Part model, mm, in its own coordinate system. A direction names the side the tool comes from. Give positions to 0.01 mm unless a question says otherwise; leave off trailing zeros. Order: outer loops, then holes, each group sorted by start corner. A loop starts at its lowest first (then second) coordinate and runs counter-clockwise, first axis right, second up.
1. Drop a flat-ended pin along its axis: pin 1 Ø0.6 at (y, z) = (-21.5, -0.5) entering from +X. Give the stop position or say it passes through.
2. Mould opens along X. For faces 4 (the cylindrical face through (-40.18, -50.29, -0.55)), 5 (the cylindrical face through (108.859, -58.797, 2.465)), 6 (the flat face through (29, 50, 2)) say: +X half, -X half, draft (parallel to the pull), parting line (faces both ways), or undercut.
3. Which spindle directions (+Z, -Z, +X, -X, +Y, -Y) get a long thin tool onto all of the face, cutting with end or side? Do faces 1 (the cylindrical face through (-39, -49.08, 0.25)), 2 (the flat face through (85, -6, 3)), 3 (the cylindrical face through (-48.797, -58.859, 2.465)). Say none if no direction does.
4. Probe line 1 (Y direction, x = -45, z = 2.7); line 2 (Y direction, x = 54.5, z = 1.15); line 3 (Y direction, x = 5.5, z = -0.2). List the from-to ranges inside material, lowest first.
5. Slice it at C-C on z = 3.6. List the corners of the cut face in (x, y), and give its area (3 significant figures).
Autodesk Fusion 360 part; units mm, degrees
sketch "Sketch2" plane through (0, 0, 0) normal (0, 0, 1) x (1, 0, 0)
  line L0 (-46, 50) -> (106, 50)
  line L1 (110, 46) -> (110, -56)
  line L2 (106, -60) -> (-46, -60)
  line L3 (-50, -56) -> (-50, 46)
  circle A0 centre (-45, 45) radius 2
  line L4 (30, -60) -> (30, 50) construction
  line L5 (-50, -5) -> (110, -5) construction
  arc A1 (-46, 50) -> (-50, 46) centre (-46, 46) ccw
  circle A2 centre (105, 45) radius 2
  arc A3 (110, 46) -> (106, 50) centre (106, 46) ccw
  circle A4 centre (105, -55) radius 2
  arc A5 (106, -60) -> (110, -56) centre (106, -56) ccw
  circle A6 centre (-45, -55) radius 2
  arc A7 (-50, -56) -> (-46, -60) centre (-46, -56) ccw
  point P0 (-50, 50)
  point P1 (110, 50)
  dimension "d3" = 4
  dimension "d4" = 5
  dimension "d5" = 5
  dimension "d6" = 4
  dimension "d63" = 160
  dimension "d64" = 110
extrude "Extrude1" add sketch "Sketch2" along normal blind 5
sketch "Sketch3" plane through (0, 0, 0) normal (0, 0, -1) x (1, 0, 0)
  circle A0 centre (105, 55) radius 2
  circle A1 centre (-45, 55) radius 2
  circle A2 centre (-45, -45) radius 2
  circle A3 centre (105, -45) radius 2
  arc A4 (-50, -46) -> (-46, -50) centre (-46, -46) ccw
  line L0 (-46, -50) -> (106, -50)
  arc A5 (106, -50) -> (110, -46) centre (106, -46) ccw
  line L1 (110, -46) -> (110, 56)
  arc A6 (110, 56) -> (106, 60) centre (106, 56) ccw
  line L2 (106, 60) -> (-46, 60)
  arc A7 (-46, 60) -> (-50, 56) centre (-46, 56) ccw
  line L3 (-50, 56) -> (-50, -46)
  line L4 (30, 60) -> (30, -50) construction
  line L5 (110, 5) -> (-50, 5) construction
  line L6 (101.7902, -41.7902) -> (-41.7901, -41.7902) construction
  line L7 (-41.7901, -41.7902) -> (-41.7901, 51.7901) construction
  line L8 (-41.7901, 51.7901) -> (101.7902, 51.7901) construction
  line L9 (101.7902, 51.7901) -> (101.7902, -41.7902) construction
  line L10 (101.7902, -41.7902) -> (-41.7901, 51.7901) construction
  line L11 (-41.7901, -41.7902) -> (101.7902, 51.7901) construction
  line L12 (95.2151, -42.8152) -> (-35.2152, -42.8152)
  line L13 (-42.8152, -35.2152) -> (-42.8152, 45.2151)
  line L14 (-35.2151, 52.8151) -> (95.2151, 52.8151)
  line L15 (102.8152, 45.2151) -> (102.8152, -35.2152)
  line L16 (88.9278, -33.6958) -> (-42.8152, 52.8151) construction
  line L17 (-37.4412, -35.28) -> (85.6746, 38.2522) construction
  line L18 (-40.7652, -35.2152) -> (-40.7652, 45.2152)
  line L19 (-35.2152, 50.7652) -> (95.2152, 50.7652)
  line L20 (100.7652, 45.2152) -> (100.7652, -35.2152)
  line L21 (98.2241, -39.1218) -> (-40.7652, 50.7652) construction
  line L22 (-34.7613, -32.5014) -> (82.9436, 35.6581) construction
  arc A8 (-35.2152, 50.7652) -> (-40.7652, 45.2152) centre (-35.2152, 45.2152) ccw
  arc A9 (-35.2151, 52.8151) -> (-42.8152, 45.2151) centre (-35.2152, 45.2151) ccw
  arc A10 (100.7652, 45.2152) -> (95.2152, 50.7652) centre (95.2152, 45.2152) ccw
  arc A11 (102.8152, 45.2151) -> (95.2151, 52.8151) centre (95.2152, 45.2151) ccw
  arc A12 (-40.7652, -35.2152) -> (-35.2152, -40.7652) centre (-35.2152, -35.2152) ccw
  arc A13 (-42.8152, -35.2152) -> (-35.2152, -42.8152) centre (-35.2152, -35.2152) ccw
  arc A14 (95.2152, -40.7652) -> (100.7652, -35.2152) centre (95.2152, -35.2152) ccw
  arc A15 (95.2151, -42.8152) -> (102.8151, -35.2152) centre (95.2151, -35.2152) ccw
  line L23 (95.2152, -40.7652) -> (-35.2152, -40.7652)
  point P0 (30, 5)
  point P1 (30, 5)
  point P2 (30, 5)
  point P3 (30, 5)
  point P4 (30, 5)
  dimension "d25" = 143.5803
  dimension "d27" = 93.5803
  dimension "d28" = 1.025
  dimension "d29" = 1.025
  dimension "d30" = 1.025
  dimension "d31" = 1.025
  dimension "d44" = 5.55
  dimension "d45" = 7.6
extrude "Extrude4" add sketch "Sketch3" along normal blind 0.8 contours L12 L13 L14 L15 A9 A11 A13 A15
draft "Draft3" angle 10 neutral plane through (0, 0, -0.8) pull (0, 0, -1) 16 faces at (8.2616, -50.7652, -0.5333) (98.4345, -49.736, -0.5333) (100.7652, -18.4051, -0.5333) (96.5236, 40.6087, -0.5333) (8.2616, 40.7652, -0.5333) (-36.2655, 40.6649, -0.5333) (-40.7652, 8.4051, -0.2667) (-39.736, -48.4345, -0.5333) (-42.8152, 8.4051, -0.5333) (-41.1892, 39.9132, -0.5333) (8.2616, 42.8152, -0.2667) (101.7969, 39.0152, -0.5333) (102.8152, -18.405, -0.5333) (97.0069, -52.6009, -0.5333) (8.2616, -52.8151, -0.2667) (-42.3972, -47.7009, -0.5333)
sketch "Sketch5" plane through (0, 0, -0.8) normal (0, 0, -1) x (1, 0, 0)
  line L0 (-35.2152, 50.7652) -> (95.2152, 50.7652)
  line L1 (100.7652, 45.2152) -> (100.7652, -35.2152)
  line L2 (95.2152, -40.7652) -> (-35.2152, -40.7652)
  line L3 (-40.7652, -35.2152) -> (-40.7652, 45.2152)
  line L4 (95.2151, 52.8151) -> (-35.2151, 52.8151)
  line L5 (-42.8152, 45.2151) -> (-42.8152, -35.2152)
  line L6 (-35.2152, -42.8152) -> (95.2151, -42.8152)
  line L7 (102.8151, -35.2152) -> (102.8152, 45.2151)
  line L8 (30, 52.8151) -> (30, -42.8152) construction
  line L9 (102.8151, 5) -> (-42.8152, 5) construction
  line L10 (101.7901, -41.7902) -> (-41.7902, -41.7902) construction
  line L11 (-41.7902, -41.7902) -> (-41.7902, 51.7901) construction
  line L12 (-41.7902, 51.7901) -> (101.7901, 51.7901) construction
  line L13 (101.7901, 51.7901) -> (101.7901, -41.7902) construction
  line L14 (101.7901, -41.7902) -> (-41.7902, 51.7901) construction
  line L15 (-41.7902, -41.7902) -> (101.7901, 51.7901) construction
  line L16 (95.2151, -42.3152) -> (-35.2151, -42.3152)
  line L17 (-42.3151, -35.2152) -> (-42.3151, 45.2151)
  line L18 (-35.2151, 52.3151) -> (95.2151, 52.3151)
  line L19 (102.3151, 45.2151) -> (102.3151, -35.2152)
  line L20 (89.0725, -33.6506) -> (-42.3151, 52.3151) construction
  line L21 (-42.3151, -42.3152) -> (89.0725, 43.6506) construction
  line L22 (95.2151, -41.2652) -> (-35.2151, -41.2652)
  line L23 (-41.2651, -35.2152) -> (-41.2651, 45.2151)
  line L24 (101.2651, 45.2151) -> (101.2651, -35.2152)
  line L25 (88.0406, -32.6798) -> (-41.2651, 51.2651) construction
  line L26 (-41.2651, -41.2652) -> (88.0406, 42.6798) construction
  arc A0 (100.7652, 45.2152) -> (95.2152, 50.7652) centre (95.2152, 45.2152) ccw
  arc A1 (95.2152, -40.7652) -> (100.7652, -35.2152) centre (95.2152, -35.2152) ccw
  arc A2 (-40.7652, -35.2152) -> (-35.2152, -40.7652) centre (-35.2152, -35.2152) ccw
  arc A3 (-35.2152, 50.7652) -> (-40.7652, 45.2152) centre (-35.2152, 45.2152) ccw
  arc A4 (-42.8152, -35.2152) -> (-35.2152, -42.8152) centre (-35.2152, -35.2152) ccw
  arc A5 (95.2151, -42.8152) -> (102.8151, -35.2152) centre (95.2152, -35.2152) ccw
  arc A6 (102.8152, 45.2151) -> (95.2151, 52.8152) centre (95.2152, 45.2152) ccw
  arc A7 (-35.2151, 52.8151) -> (-42.8151, 45.2151) centre (-35.2152, 45.2152) ccw
  arc A8 (-35.2151, 51.2651) -> (-41.2651, 45.2151) centre (-35.2151, 45.2151) ccw
  arc A9 (-35.2151, 52.3151) -> (-42.3151, 45.2151) centre (-35.2151, 45.2151) ccw
  arc A10 (101.2651, 45.2151) -> (95.2151, 51.2651) centre (95.2151, 45.2151) ccw
  arc A11 (102.3151, 45.2151) -> (95.2151, 52.3151) centre (95.2151, 45.2151) ccw
  line L27 (-35.2151, 51.2651) -> (95.2151, 51.2651)
  arc A12 (95.2151, -41.2652) -> (101.2651, -35.2152) centre (95.2151, -35.2152) ccw
  arc A13 (95.2151, -42.3152) -> (102.3151, -35.2152) centre (95.2151, -35.2152) ccw
  arc A14 (-41.2651, -35.2152) -> (-35.2151, -41.2652) centre (-35.2151, -35.2152) ccw
  arc A15 (-42.3151, -35.2152) -> (-35.2151, -42.3152) centre (-35.2151, -35.2152) ccw
  point P0 (30, 5)
  point P1 (30, 5)
  point P2 (30, 5)
  dimension "d36" = 143.5803
  dimension "d37" = 93.5803
  dimension "d38" = 0.525
  dimension "d39" = 0.525
  dimension "d40" = 0.525
  dimension "d41" = 0.525
  dimension "d50" = 6.05
  dimension "d51" = 7.1
extrude "Extrude6" cut sketch "Sketch5" against normal blind 0.5 contours L16 L17 L18 L19 A9 A11 A13 A15
extrude "Extrude7" cut 1 faces at (51.7384, -20.208, 0) along direction (0, 0, 1) blind 0.5
sketch "Sketch6" plane through (0, 0, 0.5) normal (0, 0, -1) x (1, 0, 0)
  line L0 (95.2152, 50.6241) -> (-35.2152, 50.6241)
  arc A0 (-35.2152, 50.6241) -> (-40.6241, 45.2152) centre (-35.2152, 45.2152) ccw
  line L1 (-40.6241, 45.2152) -> (-40.6241, -35.2152)
  arc A1 (-40.6241, -35.2152) -> (-35.2152, -40.6241) centre (-35.2152, -35.2152) ccw
  line L2 (-35.2152, -40.6241) -> (95.2152, -40.6241)
  arc A2 (95.2152, -40.6241) -> (100.6241, -35.2152) centre (95.2152, -35.2152) ccw
  line L3 (100.6241, -35.2152) -> (100.6241, 45.2152)
  arc A3 (100.6241, 45.2152) -> (95.2152, 50.6241) centre (95.2152, 45.2152) ccw
  line L4 (30, 50.6241) -> (30, -40.6241) construction
  line L5 (-40.6241, 5) -> (100.6241, 5) construction
  line L6 (87.5, -40) -> (-27.5, -40)
  line L7 (-27.5, -40) -> (-27.5, 50)
  line L8 (-27.5, 50) -> (87.5, 50)
  line L9 (87.5, 50) -> (87.5, -40)
  line L10 (87.5, -40) -> (-27.5, 50) construction
  line L11 (-27.5, -40) -> (87.5, 50) construction
  point P0 (30, 5)
  dimension "d58" = 115
  dimension "d59" = 90
extrude "Extrude8" cut sketch "Sketch6" against normal blind 1.1 contours L6 L7 L8 L9
sketch "Sketch7" plane through (0, 0, 1.6) normal (0, 0, -1) x (1, 0, 0)
  line L0 (87.5, 50) -> (-27.5, 50)
  line L1 (-27.5, 50) -> (-27.5, -40)
  line L2 (-27.5, -40) -> (87.5, -40)
  line L3 (87.5, -40) -> (87.5, 50)
  line L4 (30, 50) -> (30, -40) construction
  line L5 (87.5, 5) -> (-27.5, 5) construction
  line L6 (85, -37.5) -> (-25, -37.5)
  line L7 (-25, -37.5) -> (-25, 47.5)
  line L8 (-25, 47.5) -> (85, 47.5)
  line L9 (85, 47.5) -> (85, -37.5)
  line L10 (85, -37.5) -> (-25, 47.5) construction
  line L11 (-25, -37.5) -> (85, 47.5) construction
  point P0 (30, 5)
  dimension "d62" = 110
  dimension "d65" = 85
extrude "Extrude9" cut sketch "Sketch7" against normal blind 8.4 contours L6 L7 L8 L9
equation "ORingDiameter = 1 mm"
equation "ORingInnerDiameter = 150 mm"
equation "d25 = ( ORingPerimeter - 100 mm ) / 4 + 50 mm"
equation "ORingPerimeter = 2 * 3.1412 * ( ( ORingInnerDiameter / 2 ) + ORingDiameter / 2 )"
equation "d27 = ( ORingPerimeter - 100 mm ) / 4"
equation "d28 = ( ( ORingDiameter * 1.05 ) / 2 ) + 0.5 mm"
equation "d29 = ( ( ORingDiameter * 1.05 ) / 2 ) + 0.5 mm"
equation "d30 = ( ( ORingDiameter * 1.05 ) / 2 ) + 0.5 mm"
equation "d31 = ( ( ORingDiameter * 1.05 ) / 2 ) + 0.5 mm"
equation "d32 = ORingDiameter * 0.8"
equation "d36 = ( ORingPerimeter - 100 mm ) / 4 + 50 mm"
equation "d37 = ( ORingPerimeter - 100 mm ) / 4"
equation "d38 = ( ORingDiameter * 1.05 ) / 2"
equation "d39 = ( ORingDiameter * 1.05 ) / 2"
equation "d40 = ( ORingDiameter * 1.05 ) / 2"
equation "d41 = ( ORingDiameter * 1.05 ) / 2"
equation "d44 = ( ORingDiameter ) * 6 + ORingDiameter * 0.05 - 0.5 mm"
equation "d45 = ( ORingDiameter ) * 6 + ( ORingDiameter * 1.1 ) + 0.5 mm"
equation "d50 = ( ORingDiameter ) * 6 + ORingDiameter * 0.05 - 0.0 mm"
equation "d51 = ( ORingDiameter ) * 6 + ORingDiameter * 1.1 + 0 mm"
equation "PanelWidth = 90 mm"
equation "PanelLength = 115 mm"
equation "d58 = PanelLength"
equation "d59 = PanelWidth"
equation "d62 = PanelLength - 5 mm"
equation "d65 = PanelWidth - 5 mm"
Data:
1. pin 1: stops at x = 102.92
2. face 4: undercut
2. face 5: +X half
2. face 6: draft
3. face 1: -Z
3. face 2: +Z, -Z
3. face 3: +Z, -Z, -X, -Y
4. line 1: y = -60 to -57, -53 to 43, 47 to 50
4. line 2: y = -60 to -50, 40 to 50
4. line 3: y = -52.92 to -50.66, 40.66 to 42.92
5. outline: (-50, -56) arc R4 ccw to (-46, -60) - (106, -60) arc R4 ccw to (110, -56) - (110, 46) arc R4 ccw to (106, 50) - (-46, 50) arc R4 ccw to (-50, 46) - close; hole circle Ø4 at (-45, -55); hole circle Ø4 at (-45, 45); hole (-25, -47.5) - (85, -47.5) - (85, 37.5) - (-25, 37.5) - close; hole circle Ø4 at (105, -55); hole circle Ø4 at (105, 45)
5. area: 8,190 mm2
